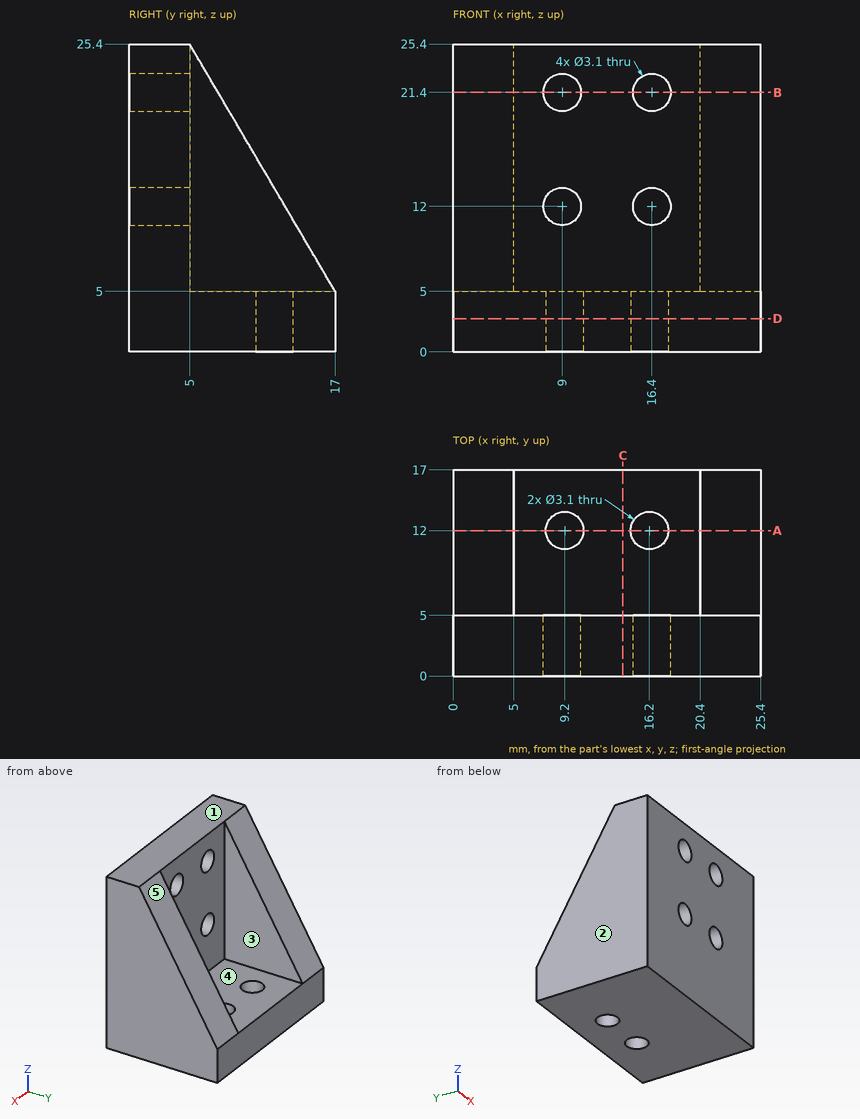
Geometry check sheet. Reference: drawing and pictorial views, mm from the part's lowest x, y, z. A direction names the side the tool comes from. Give positions to 0.01 mm unless a question says otherwise; leave off trailing zeros. Order: outer loops, then holes, each group sorted by start corner. A loop starts at its lowest first (then second) coordinate and runs counter-clockwise, first axis right, second up.
1. Section check C-C, the plane x = 14. Enter the section's corners in (y, z), and give its area (3 significant figures).
2. Section check D-D, the plane z = 2.75. Enter the section's corners in (x, y), and give its area (3 significant figures).
3. Thickness scan on L1, parallel to X at y = 3.15, z = 12; L2, parallel to X at y = 13, z = 7.5; L3, parallel to Z at x = 17.5, y = 2.75. Record the ranges inside material, lowest first.
4. Release check for a two-part mould opening along X. For the marked faces 1, 2 and 3 record: pulls with the +X half, pulls with the -X half, needs draft (parallel to the pull), parting line crosses it, or undercut.
5. Access from +Z, -Z, +X, -X, +Y, -Y to the whole of each face (thin tool, end or side, straight path). Record for the marked faces 4 and 5.
6. Gauge pin test, flat ends, axial feed: pin 1 Ø3.5 at (x, y) = (9.2, 12) entering from +Z; pin 2 Ø5 at (x, z) = (16.4, 21.4) entering from +Y; pin 3 Ø2.5 at (x, y) = (16.2, 12) entering from +Z. Record the tip position at first contact, or that the pin passes through.
7. Section check A-A, the plane y = 12. Enter the section's corners in (x, z), and give its area (3 significant figures).
8. Section check B-B, the plane z = 21.4. Enter the section's corners in (x, y).
Values follow:
1. outline: (0, 0) - (17, 0) - (17, 5) - (5, 5) - (5, 25.4) - (0, 25.4) - close
1. area: 187 mm2
2. outline: (0, 0) - (25.4, 0) - (25.4, 17) - (0, 17) - close; hole circle Ø3.1 at (9.2, 12); hole circle Ø3.1 at (16.2, 12)
2. area: 417 mm2
3. L1: x = 0 to 7.45, 10.55 to 14.85, 17.95 to 25.4
3. L2: x = 0 to 5, 20.4 to 25.4
3. L3: z = 0 to 10.91, 13.09 to 20.31, 22.49 to 25.4
4. face 1: needs draft
4. face 2: pulls with the -X half
4. face 3: undercut
5. face 4: +Z, +Y
5. face 5: +Z, +X, -X, +Y
6. pin 1: stops at z = 5
6. pin 2: stops at y = 5
6. pin 3: passes through
7. outline: (0, 0) - (7.65, 0) - (7.65, 5) - (5, 5) - (5, 13.5) - (0, 13.5) - close; (10.75, 0) - (14.65, 0) - (14.65, 5) - (10.75, 5) - close; (17.75, 0) - (25.4, 0) - (25.4, 13.5) - (20.4, 13.5) - (20.4, 5) - (17.75, 5) - close
7. area: 181 mm2
8. outline: (0, 0) - (7.45, 0) - (7.45, 5) - (5, 5) - (5, 7.35) - (0, 7.35) - close; (10.55, 0) - (14.85, 0) - (14.85, 5) - (10.55, 5) - close; (17.95, 0) - (25.4, 0) - (25.4, 7.35) - (20.4, 7.35) - (20.4, 5) - (17.95, 5) - close
